Can you work these out from the drawing? Everything is in mm from the part's minimum corner. A direction names the side the tool comes from. Coordinates: 2 decimals unless noted, no trailing zeros. Order: outer loops, then holes, each group sorted by start corner. A loop starts at its lowest first (then second) coordinate and runs counter-clockwise, first axis right, second up. Notation, with made-up numbers: (69, 85.25) -> (112, 85.25) arc R14 cw to (112, 96.25) -> close; hole circle Ø3 at (11, -27). An arc over 180 degrees is marked (long way). Use a Markdown table: item, result. Add a question column.
1) Will these pins go through, and if not, where does the flat tip stop? pin 1 Ø2 at (x, y) = (32, 23.5) entering from -Z; pin 2 Ø5 at (y, z) = (11, 66.5) entering from +X; pin 3 Ø9 at (y, z) = (21, 80) entering from -X.
2) If we section it at C-C (y = 6): Write out the boundary of the cut face in (x, z).
3) If we section it at B-B (z = 54): Write out the boundary of the cut face in (x, y).
4) If I drill on L1, parallel to X at y = 22, z = 9.5; L2, parallel to X at y = 19.5, z = 26; L3, parallel to X at y = 11.5, z = 48, over which ranges is the centre line in solid material (lowest first)? Write a range as [from, to].
5) Which directions (+Z, -Z, +X, -X, +Y, -Y) give clear straight access to the entire face, cutting with the end or side of a thin tool? Please do the marked faces 1, 2 and 3.
6) If we section it at D-D (x = 85): Write out the boundary of the cut face in (y, z).
7) If we section it at A-A (z = 11): Write out the boundary of the cut face in (x, y), plus the area to 3 significant figures.
8) Thinking about a two-plate mould opening in X: for the marked faces 4, 5 and 6, which applies, +X half, -X half, draft (parallel to the pull), parting line (faces both ways), or undercut?
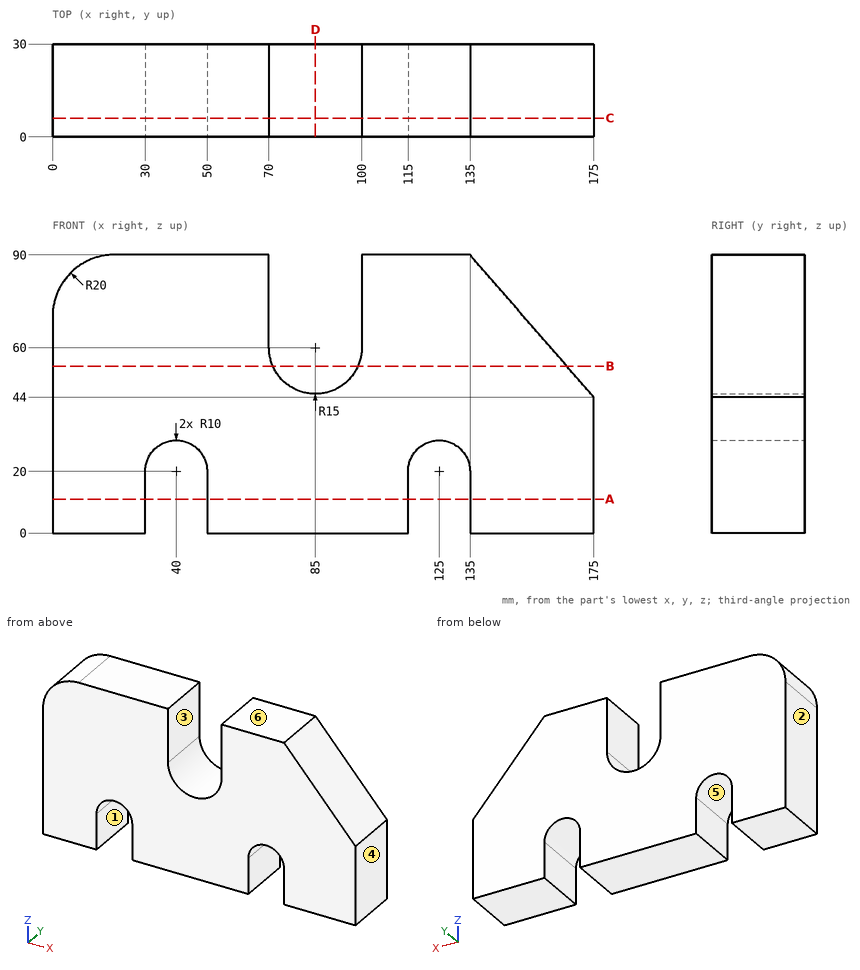
Answer sheet:
| question | item | result |
|---|---|---|
| 1 | pin 1 | z = 24.36 |
| 1 | pin 2 | x = 157.61 |
| 1 | pin 3 | x = 0.77 |
| 2 | outline | (0, 0) -> (30, 0) -> (30, 20) arc R10 cw to (50, 20) -> (50, 0) -> (115, 0) -> (115, 20) arc R10 cw to (135, 20) -> (135, 0) -> (175, 0) -> (175, 44) -> (135, 90) -> (100, 90) -> (100, 60) arc R15 cw to (70, 60) -> (70, 90) -> (20, 90) arc R20 ccw to (0, 70) -> close |
| 3 | outline | (0, 0) -> (71.25, 0) -> (71.25, 30) -> (0, 30) -> close; (98.75, 0) -> (166.3, 0) -> (166.3, 30) -> (98.75, 30) -> close |
| 4 | L1 | [0, 30], [50, 115], [135, 175] |
| 4 | L2 | [0, 32], [48, 117], [133, 175] |
| 4 | L3 | [0, 76], [94, 171.52] |
| 5 | face 1 | -Z, +Y, -Y |
| 5 | face 2 | +Z, -Z, -X, +Y, -Y |
| 5 | face 3 | +Z, +Y, -Y |
| 6 | outline | (0, 0) -> (30, 0) -> (30, 45) -> (0, 45) -> close |
| 7 | outline | (0, 0) -> (30, 0) -> (30, 30) -> (0, 30) -> close; (50, 0) -> (115, 0) -> (115, 30) -> (50, 30) -> close; (135, 0) -> (175, 0) -> (175, 30) -> (135, 30) -> close |
| 7 | area | 4,050 mm2 |
| 8 | face 4 | +X half |
| 8 | face 5 | undercut |
| 8 | face 6 | draft |
